Design review of the part built by this model. Coordinates are the model's own, in mm. A direction names the side the tool comes from. Give positions to 0.01 mm unless a question says otherwise; leave off trailing zeros. Answer as a JSON object with one key per item and string values.
Autodesk Inventor part; units mm, degrees
ref_plane "rail_to_adjusting_block_XY" through (0, 0, -67.5) normal (0, 1, 0) x (1, 0, 0)
ref_plane "rail_to_adjusting_block_YZ" through (0, 0, -67.5) normal (1, 0, 0) x (0, 0, -1)
ref_plane "rail_to_adjusting_block_ZX" through (0, 0, -67.5) normal (0, 0, -1) x (0, 1, 0)
sketch "Sketch_12" plane through (0, 0, 0) normal (0, 0, 1) x (1, 0, 0)
  line L0 (-2.5, 3.7) -> (-2.5, 3.1084)
  line L1 (-2.5, 3.1084) -> (-2.3242, 3.0098)
  arc A0 (-2.1007, 2.75) -> (-2.3242, 3.0098) centre (-2.5686, 2.5736) ccw
  line L2 (-2.1007, 2.75) -> (-1.5, 2.75)
  line L3 (-1.5, 2.75) -> (-1.5, 2.25)
  line L4 (-1.5, 2.25) -> (-2.1007, 2.25)
  arc A1 (-2.3242, 1.9902) -> (-2.1007, 2.25) centre (-2.5686, 2.4264) ccw
  line L5 (-2.3242, 1.9902) -> (-2.5, 1.8917)
  line L6 (-2.5, 1.8917) -> (-2.5, 0.3)
  line L7 (-2.5, 0.3) -> (-2.2, 0)
  line L8 (-2.2, 0) -> (2.2, 0)
  line L9 (2.2, 0) -> (2.5, 0.3)
  line L10 (2.5, 0.3) -> (2.5, 1.8917)
  line L11 (2.5, 1.8917) -> (2.3242, 1.9902)
  arc A2 (2.1007, 2.25) -> (2.3242, 1.9902) centre (2.5686, 2.4263) ccw
  line L12 (2.1007, 2.25) -> (1.5, 2.25)
  line L13 (1.5, 2.25) -> (1.5, 2.75)
  line L14 (1.5, 2.75) -> (2.1007, 2.75)
  arc A3 (2.3242, 3.0098) -> (2.1007, 2.75) centre (2.5686, 2.5737) ccw
  line L15 (2.3242, 3.0098) -> (2.5, 3.1084)
  line L16 (2.5, 3.1084) -> (2.5, 3.7)
  line L17 (2.5, 3.7) -> (2.2, 4)
  line L18 (2.2, 4) -> (-2.2, 4)
  line L19 (-2.2, 4) -> (-2.5, 3.7)
extrude "Extrusion1" add sketch "Sketch_12" along normal mid plane 145
sketch "Sketch2" plane through (-2.2, 4, 72.5) normal (0, 1, 0) x (1, 0, 0)
  point P0 (2.2, 140)
hole "Hole1" at (0, 4, -67.5) direction (0, -1, 0) diameter 2.4 depth 4 counterbore diameter 3.5 counterbore depth 1
pattern_linear "Rectangular Pattern1" count 10 spacing 15 along (0, 0, 1) of "Hole1"
ref_plane "rail_to_adjusting_block_XY" through (0, 0, -67.5) normal (0, 1, 0) x (1, 0, 0)
ref_plane "rail_to_adjusting_block_YZ" through (0, 0, -67.5) normal (1, 0, 0) x (0, 0, -1)
ref_plane "rail_to_adjusting_block_ZX" through (0, 0, -67.5) normal (0, 0, -1) x (0, 1, 0)
ref_plane "screw_1_XY" through (0, 3, 67.5) normal (0, -1, 0) x (1, 0, 0)
ref_plane "screw_1_YZ" through (0, 3, 67.5) normal (1, 0, 0) x (0, 0, 1)
ref_plane "screw_1_ZX" through (0, 3, 67.5) normal (0, 0, 1) x (0, -1, 0)
ref_plane "screw_10_XY" through (0, 3, -67.5) normal (0, -1, 0) x (1, 0, 0)
ref_plane "screw_10_YZ" through (0, 3, -67.5) normal (1, 0, 0) x (0, 0, 1)
ref_plane "screw_10_ZX" through (0, 3, -67.5) normal (0, 0, 1) x (0, -1, 0)
ref_plane "screw_2_XY" through (0, 3, 52.5) normal (0, -1, 0) x (1, 0, 0)
ref_plane "screw_2_YZ" through (0, 3, 52.5) normal (1, 0, 0) x (0, 0, 1)
ref_plane "screw_2_ZX" through (0, 3, 52.5) normal (0, 0, 1) x (0, -1, 0)
ref_plane "screw_3_XY" through (0, 3, 37.5) normal (0, -1, 0) x (1, 0, 0)
ref_plane "screw_3_YZ" through (0, 3, 37.5) normal (1, 0, 0) x (0, 0, 1)
ref_plane "screw_3_ZX" through (0, 3, 37.5) normal (0, 0, 1) x (0, -1, 0)
ref_plane "screw_4_XY" through (0, 3, 22.5) normal (0, -1, 0) x (1, 0, 0)
ref_plane "screw_4_YZ" through (0, 3, 22.5) normal (1, 0, 0) x (0, 0, 1)
ref_plane "screw_4_ZX" through (0, 3, 22.5) normal (0, 0, 1) x (0, -1, 0)
ref_plane "screw_5_XY" through (0, 3, 7.5) normal (0, -1, 0) x (1, 0, 0)
ref_plane "screw_5_YZ" through (0, 3, 7.5) normal (1, 0, 0) x (0, 0, 1)
ref_plane "screw_5_ZX" through (0, 3, 7.5) normal (0, 0, 1) x (0, -1, 0)
ref_plane "screw_6_XY" through (0, 3, -7.5) normal (0, -1, 0) x (1, 0, 0)
ref_plane "screw_6_YZ" through (0, 3, -7.5) normal (1, 0, 0) x (0, 0, 1)
ref_plane "screw_6_ZX" through (0, 3, -7.5) normal (0, 0, 1) x (0, -1, 0)
ref_plane "screw_7_XY" through (0, 3, -22.5) normal (0, -1, 0) x (1, 0, 0)
ref_plane "screw_7_YZ" through (0, 3, -22.5) normal (1, 0, 0) x (0, 0, 1)
ref_plane "screw_7_ZX" through (0, 3, -22.5) normal (0, 0, 1) x (0, -1, 0)
ref_plane "screw_8_XY" through (0, 3, -37.5) normal (0, -1, 0) x (1, 0, 0)
ref_plane "screw_8_YZ" through (0, 3, -37.5) normal (1, 0, 0) x (0, 0, 1)
ref_plane "screw_8_ZX" through (0, 3, -37.5) normal (0, 0, 1) x (0, -1, 0)
ref_plane "screw_9_XY" through (0, 3, -52.5) normal (0, -1, 0) x (1, 0, 0)
ref_plane "screw_9_YZ" through (0, 3, -52.5) normal (1, 0, 0) x (0, 0, 1)
ref_plane "screw_9_ZX" through (0, 3, -52.5) normal (0, 0, 1) x (0, -1, 0)
ref_plane "to_block_XY" through (0, 4, 36.25) normal (0, 0, 1) x (1, 0, 0)
ref_plane "to_block_YZ" through (0, 4, 36.25) normal (1, 0, 0) x (0, 1, 0)
ref_plane "to_block_ZX" through (0, 4, 36.25) normal (0, 1, 0) x (0, 0, 1)
ref_plane "to_block_2_XY" through (0, 4, -36.25) normal (0, 0, 1) x (1, 0, 0)
ref_plane "to_block_2_YZ" through (0, 4, -36.25) normal (1, 0, 0) x (0, 1, 0)
ref_plane "to_block_2_ZX" through (0, 4, -36.25) normal (0, 1, 0) x (0, 0, 1)
ref_plane "to_kue_XY" through (0, 0, 0) normal (0, 1, 0) x (1, 0, 0)
ref_plane "to_kue_YZ" through (0, 0, 0) normal (1, 0, 0) x (0, 0, -1)
ref_plane "to_kue_ZX" through (0, 0, 0) normal (0, 0, -1) x (0, 1, 0)
properties part number "SSE2B6-145_r" material "ステンレス鋼"
(1) Clearance check with flat-ended pins moving along their axes: pin 1 (1.8 mm diameter, centred on x = 0.5, z = 7, fed in from +Y); pin 2 (2 mm diameter, centred on x = 0, z = -67.5, fed in from +Y). State where each tip first meets the part, or that it passes through.
Here are the results:
{"pin 1": "stops at y = 3", "pin 2": "passes through"}
(2) For faces 1 (the flat face through (0, 3, -21)), 2 (the cylindrical face through (-0.05, 1.48, -8.7)), list the 3-axis set-ups (+Z, -Z, +X, -X, +Y, -Y) from which the entire face can be reached by the end or side of a thin tool; tool diameter is ignored.
Here are the results:
{"face 1": "+Y", "face 2": "+Y, -Y"}
(3) For line 1 along Y through (x, z) = (1.9, -28.5); line 2 along X through (y, z) = (3.7, 52.5); line 3 along X through (y, z) = (1.45, -22.5), list the stretches that pass through material, from the lowest coordinate up.
Here are the results:
{"line 1": "y = 0 to 2.25, 2.75 to 4", "line 2": "x = -2.5 to -1.75, 1.75 to 2.5", "line 3": "x = -2.5 to -1.2, 1.2 to 2.5"}
(4) We need section B-B, the plane x = 0. Give the number of separate pieces and of enclosed holes in the cut face, then the cut area to 3 significant figures.
Here are the results:
{"separate pieces": "11", "enclosed holes": "0", "area": "473 mm²"}
